Could you check a few things on this model? Use its own coordinates, in mm. A direction names the side the tool comes from. Coordinates: 2 decimals unless noted, no trailing zeros. Loops run counter-clockwise (first coordinate to the right, second up) from the corner with the lowest first, then second, coordinate; pieces in that order, holes last. Notation, with made-up numbers: M -35,60.25 L -24,60.25 A9 cw -24,71.25 Z; hole C -3.5,88.5 d3. An arc over 180 degrees is marked long. Return JSON: item names as keys, results as strings. Group by question number.
from build123d import *

# Parameters (mm, degrees)
SKETCH1_W           = 40
SKETCH1_H           = 20
BOSS_EXTRUDE1_DEPTH = 10
SKETCH2_W           = 32
SKETCH2_H           = 12
CUT_EXTRUDE1_DEPTH  = 5
FILLET1_R           = 5
SKETCH3_W           = 32
SKETCH3_H           = 12
BOSS_EXTRUDE2_DEPTH = 2.5
FILLET2_R           = 1
FILLET3_R           = 2
SMOOTHINGFILLET_R   = 0.5


with BuildPart() as part:
    # Sketch1 → Boss-Extrude1 (new body)
    with BuildSketch(Plane.XY):
        Rectangle(SKETCH1_W, SKETCH1_H)
    extrude(amount=BOSS_EXTRUDE1_DEPTH)

    # Sketch2 → Cut-Extrude1 (cut)
    with BuildSketch(Plane.XY):
        Rectangle(SKETCH2_W, SKETCH2_H)
    extrude(amount=CUT_EXTRUDE1_DEPTH, mode=Mode.SUBTRACT)

    # Fillet1
    fillet1_edges = [part.edges().sort_by_distance(p)[0] for p in [
        (-20, 0, 10),
        (0, -10, 10),
        (20, 0, 10),
        (0, 10, 10),
    ]]
    fillet(fillet1_edges, radius=FILLET1_R)

    # Sketch3 → Boss-Extrude2 (add)
    with BuildSketch(Plane.XY):
        with BuildLine():
            Line((22.5, 17.5), (-22.5, 17.5))
            ThreePointArc((-22.5, 17.5), (-24.267766953, 16.767766953), (-25, 15))
            Line((-25, 15), (-25, -15))
            ThreePointArc((-25, -15), (-24.267766953, -16.767766953), (-22.5, -17.5))
            Line((-22.5, -17.5), (22.5, -17.5))
            ThreePointArc((22.5, -17.5), (24.267766953, -16.767766953), (25, -15))
            Line((25, -15), (25, 15))
            ThreePointArc((25, 15), (24.267766953, 16.767766953), (22.5, 17.5))
        make_face()
        Rectangle(SKETCH3_W, SKETCH3_H, mode=Mode.SUBTRACT)
    extrude(amount=-BOSS_EXTRUDE2_DEPTH)

    # Fillet2
    fillet2_edges = [part.edges().sort_by_distance(p)[0] for p in [
        (16, 0, 5),
        (0, 6, 5),
        (-16, 0, 5),
        (0, -6, 5),
    ]]
    fillet(fillet2_edges, radius=FILLET2_R)

    # Fillet3
    fillet3_edges = [part.edges().sort_by_distance(p)[0] for p in [
        (0, -6, -2.5),
        (16, 0, -2.5),
        (0, 6, -2.5),
        (-16, 0, -2.5),
    ]]
    fillet(fillet3_edges, radius=FILLET3_R)

    # SmoothingFillet
    smoothingfillet_edges = [part.edges().sort_by_distance(p)[0] for p in [
        (24.267766953, 16.767766953, 0),
        (0, 17.5, 0),
        (-24.267766953, 16.767766953, 0),
        (-25, 0, 0),
        (-24.267766953, -16.767766953, 0),
        (0, -17.5, 0),
        (24.267766953, -16.767766953, 0),
        (25, 0, 0),
        (24.267766953, 16.767766953, -2.5),
        (25, 0, -2.5),
        (24.267766953, -16.767766953, -2.5),
        (0, -17.5, -2.5),
        (-24.267766953, -16.767766953, -2.5),
        (-25, 0, -2.5),
        (-24.267766953, 16.767766953, -2.5),
        (0, 17.5, -2.5),
        (0, -10, 0),
        (-20, 0, 0),
        (0, 10, 0),
        (20, 0, 0),
    ]]
    fillet(smoothingfillet_edges, radius=SMOOTHINGFILLET_R)


solid = part.part
(1) Will these pins go through, and if not, where does the flat tip stop? P1, Ø5, axis at x = 17.5, y = -6.5, coming from the -Z side; P2, Ø1.4, axis at x = -3, z = 2.5, coming from the -Y side; P3, Ø1.5, axis at y = 9, z = 3, coming from the -X side; P4, Ø5, axis at x = -7, y = 0, coming from the -Z side.
(2) Imagine slicing it at C-C, the plane x = 2. Write out the boundary of the cut face in (y, z), then the cut area to 3 significant figures.
(3) We'd pull the mould along X, two halves only. Please class faces 6 (the face through (0, -9, 8)), 7 (the face through (20, 0, 3)), 8 (the face through (0.25, -6.57, -1.9)): +X half, -X half, draft (parallel to the pull), parting line (faces both ways), or undercut.
(4) If I drill on L1, parallel to X at y = -3, z = 2; L2, parallel to Y at x = -5.5, z = 1.25; L3, parallel to Y at x = 13, z = -0.25, over which ranges is the centre line in solid material (lowest first)? Write a range as [from, to].
(5) For faces 1 (the face through (0, -10, 3)), 2 (the face through (16, 0, 2)), 3 (the face through (-24, 17, -1)), 4 (the face through (0, 10, 3)), 5 (the face through (-19, 0, 8)), which set-ups out of +Z, -Z, +X, -X, +Y, -Y let a thin tool reach every point of the face, with its end or its side?
(6) Imagine slicing it at B-B, the plane z = 2.25. Write out the boundary of the cut face in (x, y).
(7) Imagine slicing it at D-D, the plane y = -12. Write out the boundary of the cut face in (x, z).
(8) Imagine slicing it at A-A, the plane y = 4.5. Write out the boundary of the cut face in (x, z).
Checks:
{
 "1": {"P1": "z = -2.5", "P2": "y = -10", "P3": "x = -20", "P4": "z = 5"},
 "2": {"outline": "M -17.5,-2 A0.5 ccw -17,-2.5 L -8,-2.5 A2 ccw -6,-0.5 L -6,4 A1 cw -5,5 L 5,5 A1 cw 6,4 L 6,-0.5 A2 ccw 8,-2.5 L 17,-2.5 A0.5 ccw 17.5,-2 L 17.5,-0.5 A0.5 ccw 17,0 L 10.5,0 A0.5 cw 10,0.5 L 10,5 A5 ccw 5,10 L -5,10 A5 ccw -10,5 L -10,0.5 A0.5 cw -10.5,0 L -17,0 A0.5 ccw -17.5,-0.5 Z", "area": "185 mm²"},
 "3": {"face 6": "draft", "face 7": "+X half", "face 8": "undercut"},
 "4": {"L1": "[-20, -16], [16, 20]", "L2": "[-10, -6], [6, 10]", "L3": "[-17.43, -6], [6, 17.43]"},
 "5": {"face 1": "+Z, +X, -X, -Y", "face 2": "-Z", "face 3": "+Z, -Z, -X, +Y", "face 4": "+Z, +X, -X, +Y", "face 5": "+Z, -X, +Y, -Y"},
 "6": {"outline": "M -20,-10 L 20,-10 L 20,10 L -20,10 Z; hole M -16,-6 L 16,-6 L 16,6 L -16,6 Z"},
 "7": {"outline": "M -25,-2 A0.5 ccw -24.5,-2.5 L 24.5,-2.5 A0.5 ccw 25,-2 L 25,-0.5 A0.5 ccw 24.5,0 L -24.5,0 A0.5 ccw -25,-0.5 Z"},
 "8": {"outline": "M -25,-2 A0.5 ccw -24.5,-2.5 L -18,-2.5 A2 ccw -16,-0.5 L -16,4 A1 cw -15,5 L 15,5 A1 cw 16,4 L 16,-0.5 A2 ccw 18,-2.5 L 24.5,-2.5 A0.5 ccw 25,-2 L 25,-0.5 A0.5 ccw 24.5,0 L 20.5,0 A0.5 cw 20,0.5 L 20,5 A5 ccw 15,10 L -15,10 A5 ccw -20,5 L -20,0.5 A0.5 cw -20.5,0 L -24.5,0 A0.5 ccw -25,-0.5 Z"}
}
